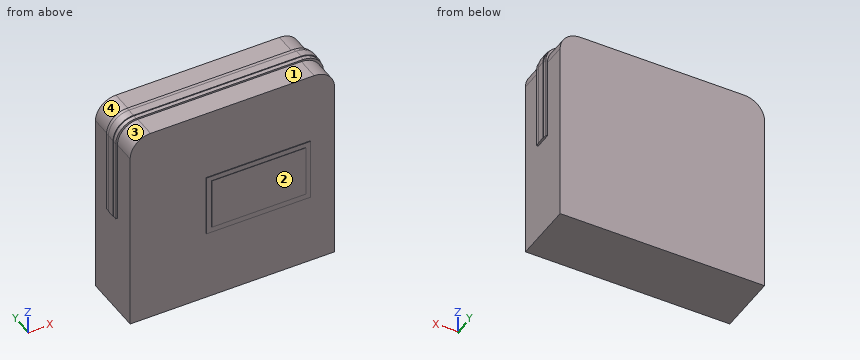
from build123d import *

# Parameters (mm, degrees)
F0_W      = 250
F0_H      = 75
F2_DEPTH  = 125
F1_W      = 254
F1_H      = 20
F3_DEPTH  = 127
F4_R      = 25
F5_W      = 255
F5_H      = 10
F6_DEPTH  = 128
F7_R      = 25
F8_W      = 127
F8_H      = 76
F9_DEPTH  = 1
F11_DEPTH = 0.6


with BuildPart() as f2:
    # F0 (on Top) → F2 (new body, symmetric)
    with BuildSketch(Plane.XY):
        Rectangle(F0_W, F0_H)
    extrude(amount=F2_DEPTH, both=True)

    # F1 (on Top) → F3 (join)
    with BuildSketch(Plane.XY):
        Rectangle(F1_W, F1_H)
    extrude(amount=F3_DEPTH)

    # F4
    f4_edges = [f2.edges().sort_by_distance(p)[0] for p in [
        (-127, 0, 127),
        (-125, 23.75, 125),
        (-125, -23.75, 125),
        (125, 23.75, 125),
        (125, -23.75, 125),
        (127, 0, 127),
    ]]
    fillet(f4_edges, radius=F4_R)

    # F5 (on Top) → F6 (join)
    with BuildSketch(Plane.XY):
        Rectangle(F5_W, F5_H)
    extrude(amount=F6_DEPTH)

    # F7
    f7_edges = [f2.edges().sort_by_distance(p)[0] for p in [
        (-127.5, 0, 128),
        (127.5, 0, 128),
    ]]
    fillet(f7_edges, radius=F7_R)

    # F8 (on face) → F9 (join)
    with BuildSketch(Plane.XZ.offset(37.5)):
        with Locations((31.5, 0)):
            Rectangle(F8_W, F8_H)
    extrude(amount=F9_DEPTH)

    # F10 (on face) → F11 (join)
    with BuildSketch(Plane.XZ.offset(38.5)):
        Polygon((-26, 32), (-26, -31), (89, -31), (89, 32), (76.5, 26), (-13.5, 26), align=None)
        Polygon((89, 32), (-26, 32), (-13.5, 26), (76.5, 26), align=None)
    extrude(amount=F11_DEPTH)


solid = f2.part
Check sheet for the modelled part. Datum: model origin and axes. Units: mm. Face numbers are marked on the shaded views. A direction names the side the tool comes from. Round coordinates to 2 decimals unless told otherwise and drop trailing zeros. Loops run counter-clockwise (first coordinate to the right, second up) from the corner with the lowest first, then second, coordinate; pieces in that order, holes last.
1. Sectioned sample at D-D on x = 75. Record the boundary of the cut face in (y, z), and give its area (3 significant figures).
2. Scan lines: probe 1 along Z at (x, y) = (51.5, 18); probe 2 along Y at (x, z) = (76, -100). Record each from-to range of solid material in increasing order.
3. Gauge pin test, flat ends, axial feed: pin 1 Ø1.5 at (y, z) = (8.5, 59) entering from -X; pin 2 Ø6 at (x, z) = (-76, -28) entering from -Y; pin 3 Ø3 at (y, z) = (29, 92.5) entering from -X. Record the tip position at first contact, or that the pin passes through.
4. Set-up check for the marked faces 1, 2, 3 and 4: record each of +Z, -Z, +X, -X, +Y, -Y from which the full face is reachable in a straight line by a thin tool's end or side.
5. Sectioned sample at B-B on y = -20. Record the boundary of the cut face in (x, z).
6. Sectioned sample at A-A on x = -47. Record the boundary of the cut face in (y, z), and give its area (3 significant figures).
7. Sectioned sample at C-C on z = 86.5. Record the boundary of the cut face in (x, y).
Recorded:
1. outline: (-39.1, -31) - (-38.5, -31) - (-38.5, -38) - (-37.5, -38) - (-37.5, -125) - (37.5, -125) - (37.5, 125) - (10, 125) - (10, 127) - (5, 127) - (5, 128) - (-5, 128) - (-5, 127) - (-10, 127) - (-10, 125) - (-37.5, 125) - (-37.5, 38) - (-38.5, 38) - (-38.5, 32) - (-39.1, 32) - close
1. area: 18,900 mm2
2. probe 1: z = -125 to 125
2. probe 2: y = -37.5 to 37.5
3. pin 1: stops at x = -127
3. pin 2: stops at y = -37.5
3. pin 3: stops at x = -125
4. face 1: +Z, +X, -X, -Y
4. face 2: +Z, -Z, +X, -X, -Y
4. face 3: +Z, -X, -Y
4. face 4: +Z, -X, +Y
5. outline: (-125, -125) - (125, -125) - (125, 100) arc R25 ccw to (100, 125) - (-100, 125) arc R25 ccw to (-125, 100) - close
6. outline: (-37.5, -125) - (37.5, -125) - (37.5, 125) - (10, 125) - (10, 127) - (5, 127) - (5, 128) - (-5, 128) - (-5, 127) - (-10, 127) - (-10, 125) - (-37.5, 125) - close
6. area: 18,800 mm2
7. outline: (-127.5, -5) - (-127, -5) - (-127, -10) - (-125, -10) - (-125, -37.5) - (125, -37.5) - (125, -10) - (127, -10) - (127, -5) - (127.5, -5) - (127.5, 5) - (127, 5) - (127, 10) - (125, 10) - (125, 37.5) - (-125, 37.5) - (-125, 10) - (-127, 10) - (-127, 5) - (-127.5, 5) - close
